CAD build for the part. Positions are in the model's coordinates, mm. Round coordinates to 2 decimals unless told otherwise and drop trailing zeros. Order: outer loops, then holes, each group sorted by start corner. A loop starts at its lowest first (then second) coordinate and runs counter-clockwise, first axis right, second up.
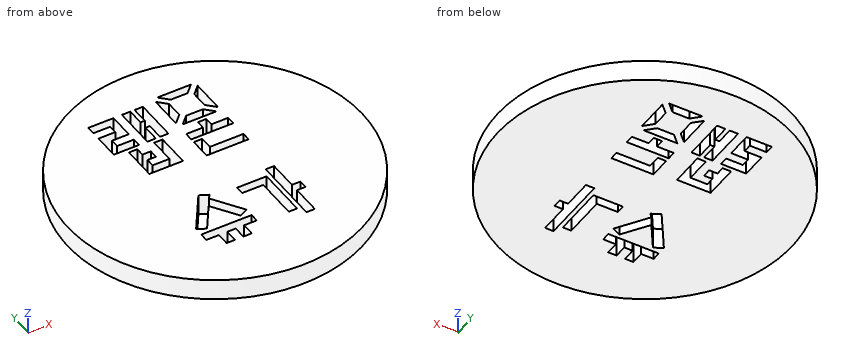
```python
from build123d import *

# Parameters (mm, degrees)
F0_R     = 35
F1_DEPTH = 5


with BuildPart() as f1:
    # F0 (on Top) → F1 (new body)
    with BuildSketch(Plane.XY):
        with Locations((-51.047989, -3.453226)):
            Circle(F0_R)
        Polygon((-59.047989, -24.453226), (-61.047989, -24.453226), (-61.047989, -21.453226), (-64.047989, -21.453226), (-64.047989, -19.453226), (-52.047989, -19.453226), (-52.047989, -21.453226), (-55.047989, -21.453226), (-55.047989, -24.453226), (-57.047989, -24.453226), (-57.047989, -21.453226), (-59.047989, -21.453226), align=None, mode=Mode.SUBTRACT)
        Polygon((-64.047989, -17.453226), (-58.047989, -8.45281), (-56.047989, -9.452658), (-56.714722, -10.452803), (-52.047989, -17.453226), (-54.047989, -18.453125), (-58.047951, -12.45274), (-62.047989, -18.453074), align=None, mode=Mode.SUBTRACT)
        Polygon((-43.047989, -10.453226), (-43.047989, -22.453226), (-45.047989, -22.453226), (-45.047989, -12.453226), (-50.047989, -12.453226), (-50.047989, -10.453226), align=None, mode=Mode.SUBTRACT)
        Polygon((-42.047989, -8.453226), (-40.047989, -8.453226), (-40.047989, -15.453226), (-38.047989, -15.453226), (-38.047989, -17.453226), (-40.047989, -17.453226), (-40.047989, -24.453226), (-42.047989, -24.453226), (-42.047989, -22.453226), align=None, mode=Mode.SUBTRACT)
        Polygon((-57.047989, 10.546774), (-55.047989, 10.546774), (-55.047989, 2.546774), (-63.047989, 2.546774), (-63.047989, 10.546774), (-61.047989, 10.546774), (-61.047989, 8.546774), (-59.047989, 8.546774), (-59.047989, 6.546774), (-61.047989, 6.546774), (-61.047989, 4.546774), (-57.047989, 4.546774), align=None, mode=Mode.SUBTRACT)
        Polygon((-66.047989, 19.546774), (-66.047989, 21.546774), (-60.047989, 21.546774), (-60.047989, 15.546774), (-64.047989, 15.546774), (-64.047989, 13.546774), (-60.047989, 13.546774), (-60.047989, 11.546774), (-66.047989, 11.546774), (-66.047989, 17.546774), (-62.047989, 17.546774), (-62.047989, 19.546774), align=None, mode=Mode.SUBTRACT)
        Polygon((-58.047989, 11.546774), (-58.047989, 21.546774), (-56.047989, 21.546774), (-56.047989, 17.546774), (-55.047989, 17.546774), (-55.047989, 21.546774), (-53.047989, 21.546774), (-53.047989, 11.546774), (-55.047989, 11.546774), (-55.047989, 15.546774), (-56.047989, 15.546774), (-56.047989, 11.546774), align=None, mode=Mode.SUBTRACT)
        Polygon((-50.047989, 1.546774), (-50.047989, 6.546774), (-48.047989, 6.546774), (-48.047989, 3.546774), (-40.047989, 3.546774), (-40.047989, 1.546774), align=None, mode=Mode.SUBTRACT)
        Polygon((-44.047989, 9.547076), (-40.047989, 9.547076), (-40.047989, 7.547076), (-50.047989, 7.547076), (-50.047989, 9.547076), (-46.047989, 9.547076), (-46.047989, 11.547076), (-44.047989, 11.547076), align=None, mode=Mode.SUBTRACT)
        Polygon((-43.048291, 14.546774), (-41.047536, 12.548133), (-49.04814, 12.546925), (-47.048593, 14.546774), align=None, mode=Mode.SUBTRACT)
        Polygon((-48.048291, 19.547076), (-48.048291, 15.546472), (-50.047989, 13.546774), (-50.047989, 21.546774), align=None, mode=Mode.SUBTRACT)
        Polygon((-47.047989, 20.546774), (-49.048593, 22.546774), (-41.047989, 22.546774), (-43.047385, 20.546774), align=None, mode=Mode.SUBTRACT)
        Polygon((-40.048593, 13.546774), (-42.048291, 15.546472), (-42.048291, 19.547076), (-40.048593, 21.546774), align=None, mode=Mode.SUBTRACT)
    extrude(amount=F1_DEPTH)


solid = f1.part
```
1. Cut at B-B, the plane x = -37. Write the cut outline in (y, z), and give its area (3 significant figures).
2. Cut at A-A, the plane y = 16.5. Write the cut outline in (x, z), and give its area (3 significant figures).
3. Cut at D-D, the plane z = 3.6. Give the number of separate pieces and of enclosed holes in the cut face, and give its area (3 significant figures).
4. Pin check, flat tips, straight feed: P1, Ø2.5, axis at y = -22.5, z = 3.5, coming from the +X side; P2, Ø2, axis at x = -47.5, y = 3.5, coming from the +Z side; P3, Ø1.6, axis at x = -45, z = 1.5, coming from the -Y side; P4, Ø1.5, axis at x = -71.5, z = 0.5, coming from the -Y side. Stop position of each tip, or through.
5. Cut at C-C, the plane y = 25.5. Write the cut outline in (x, z).
6. Drill centre lines: line 1 (X direction, y = -20, z = 1.9); line 2 (X direction, y = -23, z = 0.4); line 3 (Y direction, x = -59, z = 2.85). Where is each one in solid material? Low to high.
Outcome:
1. outline: (-35.51, 0) - (28.6, 0) - (28.6, 5) - (-35.51, 5) - close
1. area: 321 mm2
2. outline: (-79.8, 0) - (-66.05, 0) - (-66.05, 5) - (-79.8, 5) - close; (-60.05, 0) - (-58.05, 0) - (-58.05, 5) - (-60.05, 5) - close; (-53.05, 0) - (-50.05, 0) - (-50.05, 5) - (-53.05, 5) - close; (-48.05, 0) - (-42.05, 0) - (-42.05, 5) - (-48.05, 5) - close; (-40.05, 0) - (-22.29, 0) - (-22.29, 5) - (-40.05, 5) - close
2. area: 213 mm2
3. separate pieces: 1
3. enclosed holes: 13
3. area: 3,470 mm2
4. P1: stops at x = -20.91
4. P2: stops at z = 5
4. P3: stops at y = -38.06
4. P4: stops at y = -32.38
5. outline: (-70.71, 0) - (-31.38, 0) - (-31.38, 5) - (-70.71, 5) - close
6. line 1: x = -81.89 to -64.05, -52.05 to -45.05, -43.05 to -42.05, -40.05 to -20.21
6. line 2: x = -80.08 to -61.05, -59.05 to -57.05, -55.05 to -42.05, -40.05 to -22.01
6. line 3: y = -37.54 to -21.45, -19.45 to -13.88, -9.88 to 2.55, 4.55 to 30.63
